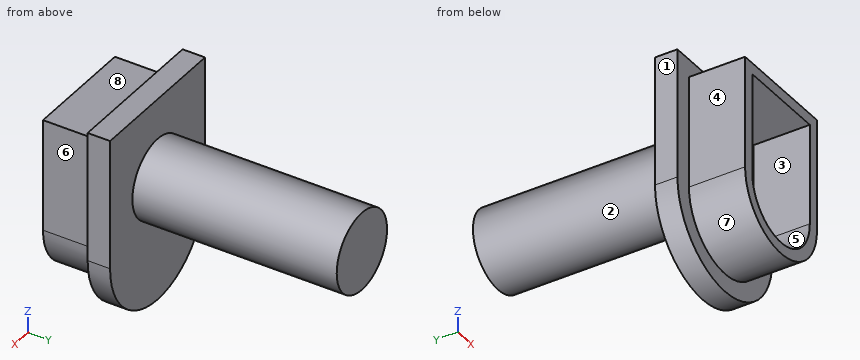
from build123d import *

# Parameters (mm, degrees)
F0_R     = 3.5
F1_DEPTH = 2
F2_DEPTH = 5
F3_DEPTH = 20.2


with BuildPart() as f1:
    # F0 (on Front) → F1 (new body)
    with BuildSketch(Plane.XZ):
        with BuildLine():
            Line((-12.4122027444, 20.418163389), (-25.6122041357, 20.418163389))
            Line((-25.6122041357, 20.418163389), (-25.6122041357, 8.8181626933))
            ThreePointArc((-25.6122041357, 8.8181626933), (-19.0122034401, 2.2181619977), (-12.4122027444, 8.8181626933))
            Line((-12.4122027444, 8.8181626933), (-12.4122027444, 20.418163389))
        make_face()
        with BuildLine():
            Line((-24.0122034401, 8.8181626933), (-24.0122034401, 18.8181626933))
            Line((-24.0122034401, 18.8181626933), (-14.0122034401, 18.8181626933))
            Line((-14.0122034401, 18.8181626933), (-14.0122034401, 8.8181626933))
            ThreePointArc((-14.0122034401, 8.8181626933), (-19.0122034401, 3.8181626933), (-24.0122034401, 8.8181626933))
        make_face(mode=Mode.SUBTRACT)
        with BuildLine():
            Line((-14.0122034401, 18.8181626933), (-24.0122034401, 18.8181626933))
            Line((-24.0122034401, 18.8181626933), (-24.0122034401, 8.8181626933))
            ThreePointArc((-24.0122034401, 8.8181626933), (-19.0122034401, 3.8181626933), (-14.0122034401, 8.8181626933))
            Line((-14.0122034401, 8.8181626933), (-14.0122034401, 18.8181626933))
        make_face()
        with BuildLine():
            Line((-23.0122034401, 8.8181626933), (-23.0122034401, 17.8181626933))
            Line((-23.0122034401, 17.8181626933), (-15.0122034401, 17.8181626933))
            Line((-15.0122034401, 17.8181626933), (-15.0122034401, 8.8181626933))
            ThreePointArc((-15.0122034401, 8.8181626933), (-19.0122034401, 4.8181626933), (-23.0122034401, 8.8181626933))
        make_face(mode=Mode.SUBTRACT)
        with BuildLine():
            Line((-15.0122034401, 17.8181626933), (-23.0122034401, 17.8181626933))
            Line((-23.0122034401, 17.8181626933), (-23.0122034401, 8.8181626933))
            ThreePointArc((-23.0122034401, 8.8181626933), (-19.0122034401, 4.8181626933), (-15.0122034401, 8.8181626933))
            Line((-15.0122034401, 8.8181626933), (-15.0122034401, 17.8181626933))
        make_face()
        with Locations((-19.0122034401, 13.3181626933)):
            Circle(F0_R, mode=Mode.SUBTRACT)
    extrude(amount=-F1_DEPTH)

    # F0 (on Front) → F2 (join)
    with BuildSketch(Plane.XZ):
        with BuildLine():
            Line((-14.0122034401, 18.8181626933), (-24.0122034401, 18.8181626933))
            Line((-24.0122034401, 18.8181626933), (-24.0122034401, 8.8181626933))
            ThreePointArc((-24.0122034401, 8.8181626933), (-19.0122034401, 3.8181626933), (-14.0122034401, 8.8181626933))
            Line((-14.0122034401, 8.8181626933), (-14.0122034401, 18.8181626933))
        make_face()
        with BuildLine():
            Line((-23.0122034401, 8.8181626933), (-23.0122034401, 17.8181626933))
            Line((-23.0122034401, 17.8181626933), (-15.0122034401, 17.8181626933))
            Line((-15.0122034401, 17.8181626933), (-15.0122034401, 8.8181626933))
            ThreePointArc((-15.0122034401, 8.8181626933), (-19.0122034401, 4.8181626933), (-23.0122034401, 8.8181626933))
        make_face(mode=Mode.SUBTRACT)
    extrude(amount=F2_DEPTH)

    # F0 (on Front) → F3 (join)
    with BuildSketch(Plane.XZ):
        with Locations((-19.0122034401, 13.3181626933)):
            Circle(F0_R)
    extrude(amount=-F3_DEPTH)


solid = f1.part
The listing builds one solid part. Answer for the finished solid, in the listing's coordinates (mm). Face numbers are marked on the shaded views. A direction names the side the tool comes from. Give positions to 0.01 mm unless a question says otherwise; leave off trailing zeros. Write each loop counter-clockwise with the first axis right and the second up, starting at its lowest first coordinate (ties: lowest second). Pieces come first, ordered by that corner, then holes.
1) Section C-C (z = 14) is taken. Write down the section's boundary in (x, y), and give its area (3 significant figures).
2) Find the intervals of material crossed by L1, parallel to X at y = -3.5, z = 16.25; L2, parallel to Y at x = -19.25, z = 17.5; L3, parallel to Z at x = -19, y = 2.5, in increasing order.
3) A tool of negligible diameter and unlimited length cuts with its end or side. For the marked faces 4, 5, 6, 7 and 8, from which of +Z, -Z, +X, -X, +Y, -Y can it reach the whole face along a straight path? Write none if from no direction.
4) Section A-A (y = -2.75) is taken. Write down the section's boundary in (x, z).
5) Given P1, Ø5.5, axis at y = -3.5, z = 13.5, coming from the -X side; P2, Ø2.5, axis at x = -20, y = -3, coming from the +Z side; P3, Ø6, axis at y = 7.5, z = 7.5, coming from the +X side, each flat-ended and moving along its own axis, determine where each tip first touches the part or whether it passes through.
6) For a pull along Z with two mould halves and no side action, classify the marked faces 1, 2 and 3 as pulls with the +Z half, pulls with the -Z half, needs draft (parallel to the pull), parting line crosses it, or undercut.
7) Section D-D (y = 1) is taken. Write down the section's boundary in (x, z).
8) Section B-B (x = -18.75) is taken. Write down the section's boundary in (y, z), and give its area (3 significant figures).
Response:
1. outline: (-25.61, 0) - (-24.01, 0) - (-24.01, -5) - (-23.01, -5) - (-23.01, 0) - (-15.01, 0) - (-15.01, -5) - (-14.01, -5) - (-14.01, 0) - (-12.41, 0) - (-12.41, 2) - (-15.58, 2) - (-15.58, 20.2) - (-22.45, 20.2) - (-22.45, 2) - (-25.61, 2) - close
1. area: 161 mm2
2. L1: x = -24.01 to -23.01, -15.01 to -14.01
2. L2: y = 0 to 2
2. L3: z = 9.82 to 16.82
3. face 4: +Z, -Z, -X, -Y
3. face 5: -Y
3. face 6: +Z, -Z, +X, -Y
3. face 7: -Z, -Y
3. face 8: +Z, +X, -X, -Y
4. outline: (-24.01, 8.82) arc R5 ccw to (-14.01, 8.82) - (-14.01, 18.82) - (-24.01, 18.82) - close; hole (-23.01, 8.82) arc R4 ccw to (-15.01, 8.82) - (-15.01, 17.82) - (-23.01, 17.82) - close
5. P1: stops at x = -24.01
5. P2: stops at z = 18.82
5. P3: stops at x = -16.94
6. face 1: needs draft
6. face 2: parting line crosses it
6. face 3: undercut
7. outline: (-25.61, 8.82) arc R6.6 ccw to (-12.41, 8.82) - (-12.41, 20.42) - (-25.61, 20.42) - close
8. outline: (-5, 3.83) - (0, 3.83) - (0, 2.22) - (2, 2.22) - (2, 9.83) - (20.2, 9.83) - (20.2, 16.81) - (2, 16.81) - (2, 20.42) - (0, 20.42) - (0, 18.82) - (-5, 18.82) - (-5, 17.82) - (0, 17.82) - (0, 4.83) - (-5, 4.83) - close
8. area: 173 mm2
